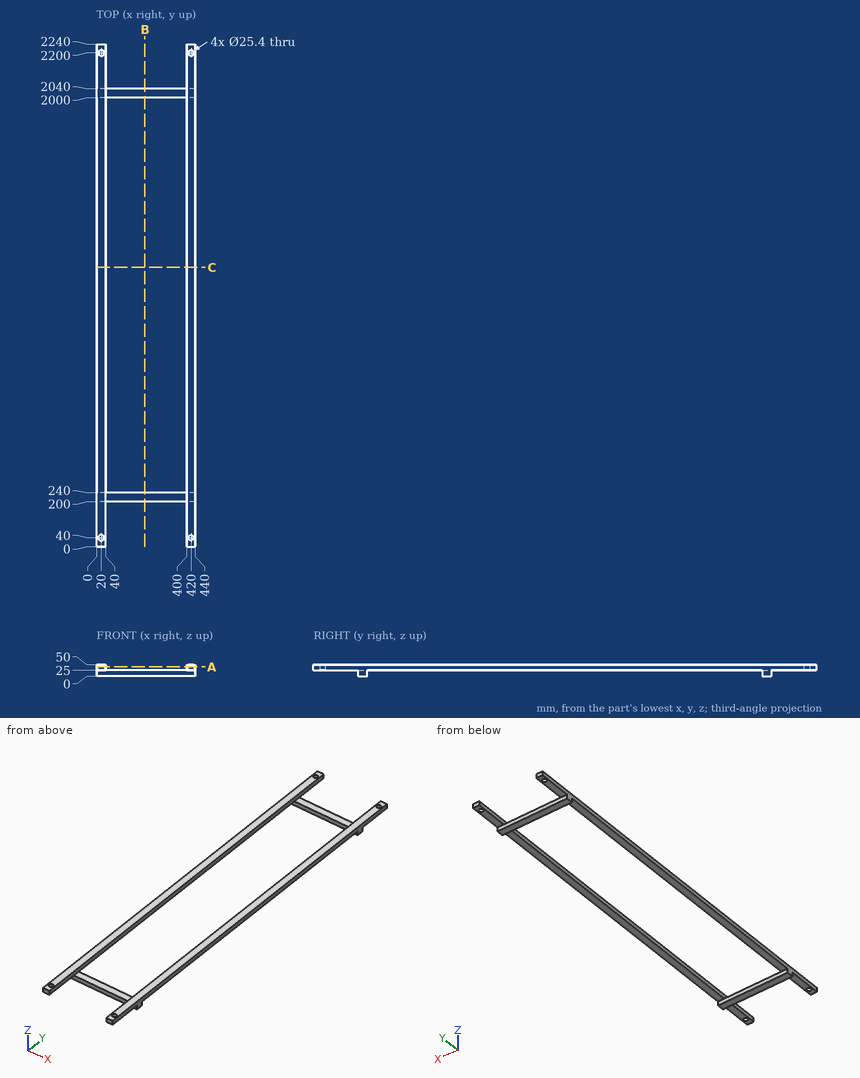
Can you work these out from the drawing? Everything is in mm from the part's minimum corner. Round coordinates to 2 decimals unless told otherwise and drop trailing zeros. Write each loop counter-clockwise with the first axis right and the second up, starting at its lowest first coordinate (ties: lowest second). Pieces come first, ordered by that corner, then holes.
1. Suppose I cut it at A-A (z = 41). List the corners of the cut face in (x, y) for me, and give its area (3 significant figures).
2. Suppose I cut it at B-B (x = 214). List the corners of the cut face in (y, z) for me, and give its area (3 significant figures).
3. Suppose I cut it at C-C (y = 1244.5). List the corners of the cut face in (x, z) for me.
4. Will these pins go through, and if not, where does the flat tip stop? pin 1 Ø20 at (x, z) = (114.5, 17.5) entering from +Y; pin 2 Ø12 at (x, y) = (19.5, 1330.5) entering from -Z; pin 3 Ø3 at (x, z) = (300, 15.5) entering from -Y.
5. I need wall thicknesses on L1, parallel to Y at x = 420, z = 40.25; L2, parallel to X at y = 40, z = 43; L3, parallel to X at y = 794, z = 47. Which ranges of each line are inside material? Lowest first, please.
Answer sheet:
1. outline: (0, 0) - (40, 0) - (40, 2240) - (0, 2240) - close; (400, 0) - (440, 0) - (440, 2240) - (400, 2240) - close; hole circle Ø25.4 at (20, 40); hole circle Ø25.4 at (20, 2200); hole circle Ø25.4 at (420, 40); hole circle Ø25.4 at (420, 2200)
1. area: 177,000 mm2
2. outline: (200, 0) - (240, 0) - (240, 25) - (200, 25) - close; (2000, 0) - (2040, 0) - (2040, 25) - (2000, 25) - close
2. area: 2,000 mm2
3. outline: (0, 25) - (40, 25) - (40, 50) - (0, 50) - close; (400, 25) - (440, 25) - (440, 50) - (400, 50) - close
4. pin 1: stops at y = 2040
4. pin 2: stops at z = 25
4. pin 3: stops at y = 200
5. L1: y = 0 to 27.3, 52.7 to 2187.3, 2212.7 to 2240
5. L2: x = 0 to 7.3, 32.7 to 40, 400 to 407.3, 432.7 to 440
5. L3: x = 0 to 40, 400 to 440
